from build123d import *

# Parameters (mm, degrees)
SKETCH_1_R      = 3.4
SKETCH_1_R_2    = 2.25
EXTRUDE_1_DEPTH = 4.85
EXTRUDE_START   = 0.5
SKETCH_2_R      = 2.25
SKETCH_2_R_2    = 0.5
EXTRUDE_2_DEPTH = 2
EXTRUDE_START_2 = 1.25
SKETCH_3_R      = 2.25
SKETCH_3_R_2    = 1.15
EXTRUDE_3_DEPTH = 0.9


with BuildPart() as part:
    # 草图1 → 凸台-拉伸1 (new body)
    with BuildSketch(Plane(origin=(0, 0, 0), x_dir=(1, 0, 0), z_dir=(0, 1, 0))):
        with Locations(Location((0, 0, 0), (0, 0, 270))):
            Circle(SKETCH_1_R)
        with Locations(Location((0, 0, 0), (0, 0, 270))):
            Circle(SKETCH_1_R_2, mode=Mode.SUBTRACT)
    extrude(amount=EXTRUDE_1_DEPTH)

    # 草图2 → 凸台-拉伸2 (add)
    with BuildSketch(Plane(origin=(0, 0, 0), x_dir=(1, 0, 0), z_dir=(0, 1, 0)).offset(EXTRUDE_START)):
        with BuildLine():
            Line((1.781000011, 3.395903963), (1.781000011, 6.35))
            ThreePointArc((1.781000011, 6.35), (0, 8.13100001), (-1.781000011, 6.35))
            Line((-1.781000011, 6.35), (-1.781000011, 3.342130588))
            ThreePointArc((-1.781000011, 3.342130588), (-3.786362647, -0.072496957), (-1.651758938, -3.407857144))
            Line((-1.651758938, -3.407857144), (-1.651758938, -6.35))
            ThreePointArc((-1.651758938, -6.35), (0, -8.001758939), (1.651758938, -6.35))
            Line((1.651758938, -6.35), (1.651758938, -3.407857144))
            Line((1.651758938, -3.407857144), (15.410111856, -2.130295801))
            ThreePointArc((15.410111856, -2.130295801), (17.490132215, -0.073847388), (15.557558889, 2.121744812))
            Line((15.557558889, 2.121744812), (1.781000011, 3.395903963))
        make_face()
        with Locations(Location((0, 0, 0), (0, 0, 270))):
            Circle(SKETCH_2_R, mode=Mode.SUBTRACT)
        with Locations(Location((0, -6.75, 0), (0, 0, 270))):
            Circle(SKETCH_2_R_2, mode=Mode.SUBTRACT)
        with Locations(Location((0, -4.75, 0), (0, 0, 270))):
            Circle(SKETCH_2_R_2, mode=Mode.SUBTRACT)
        with Locations(Location((15, 0, 0), (0, 0, 270))):
            Circle(SKETCH_2_R_2, mode=Mode.SUBTRACT)
        with Locations(Location((13, 0, 0), (0, 0, 270))):
            Circle(SKETCH_2_R_2, mode=Mode.SUBTRACT)
        with Locations(Location((11, 0, 0), (0, 0, 270))):
            Circle(SKETCH_2_R_2, mode=Mode.SUBTRACT)
        with Locations(Location((9, 0, 0), (0, 0, 270))):
            Circle(SKETCH_2_R_2, mode=Mode.SUBTRACT)
        with Locations(Location((7, 0, 0), (0, 0, 270))):
            Circle(SKETCH_2_R_2, mode=Mode.SUBTRACT)
        with Locations(Location((5, 0, 0), (0, 0, 270))):
            Circle(SKETCH_2_R_2, mode=Mode.SUBTRACT)
        with Locations(Location((0, 6.75, 0), (0, 0, 270))):
            Circle(SKETCH_2_R_2, mode=Mode.SUBTRACT)
        with Locations(Location((0, 4.75, 0), (0, 0, 270))):
            Circle(SKETCH_2_R_2, mode=Mode.SUBTRACT)
    extrude(amount=EXTRUDE_2_DEPTH)

    # 草图3 → 凸台-拉伸3 (add)
    with BuildSketch(Plane(origin=(0, 0, 0), x_dir=(1, 0, 0), z_dir=(0, 1, 0)).offset(EXTRUDE_START_2)):
        with Locations(Location((0, 0, 0), (0, 0, 270))):
            Circle(SKETCH_3_R)
        with Locations(Location((0, 0, 0), (0, 0, 270))):
            Circle(SKETCH_3_R_2, mode=Mode.SUBTRACT)
    extrude(amount=EXTRUDE_3_DEPTH)


solid = part.part
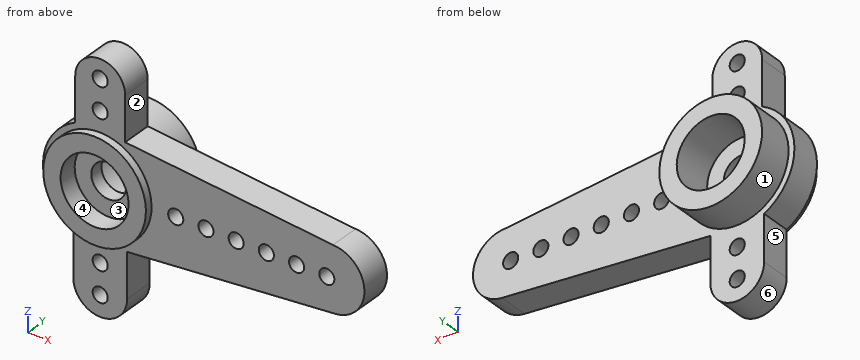
The listing builds one solid part. Answer for the finished solid, in the listing's coordinates (mm). Face numbers are marked on the shaded views. A direction names the side the tool comes from. Give positions to 0.01 mm unless a question says otherwise; leave off trailing zeros. Write each loop counter-clockwise with the first axis right and the second up, starting at its lowest first coordinate (ties: lowest second). Pieces come first, ordered by that corner, then holes. Notation, with made-up numbers: (1, 15.5) - (34, 15.5) arc R25 cw to (34, 32.5) - close; hole circle Ø3 at (39.25, -27). An arc over 180 degrees is marked (long way). Use a Markdown table: item, result.
1. Section C-C on y = 4.3 is taken. Write down the section's boundary in (x, z).
Values follow:
| item | result |
|---|---|
| outline | circle Ø6.8 at (0, 0); hole circle Ø4.5 at (0, 0) |
2. For a pull along X with two mould halves and no side action, classify the marked faces 4, 5 and 6 as released by +X, released by -X, zero draft, split by the parting line, or undercut.
Values follow:
| item | result |
|---|---|
| face 4 | undercut |
| face 5 | released by -X |
| face 6 | split by the parting line |
3. Section D-D on z = -2.75 is taken. Write down the section's boundary in (x, y).
Values follow:
| item | result |
|---|---|
| outline | (-2.6, 0.5) - (-2, 0.5) - (-2, 0) - (2, 0) - (2, 0.5) - (8.76, 0.5) - (8.76, 2.5) - (2, 2.5) - (2, 4.85) - (-2, 4.85) - (-2, 2.5) - (-2.6, 2.5) - close |
4. Find the intervals of material crossed by probe 1 along Y at (x, z) = (16.75, -1.5); probe 2 along X at (y, z) = (2.05, 4.75); probe 3 along X at (y, z) = (1, -4.75), in increasing order. Write a range as from..to.
Values follow:
| item | result |
|---|---|
| probe 1 | y = 0.5..2.5 |
| probe 2 | x = -1.65..-0.5, 0.5..1.65 |
| probe 3 | x = -1.78..-0.5, 0.5..1.78 |
5. Section A-A on z = 4.75 is taken. Write down the section's boundary in (x, y), plus the area to 3 significant figures.
Values follow:
| item | result |
|---|---|
| outline | (-1.65, 0.5) - (-0.5, 0.5) - (-0.5, 2.5) - (-1.65, 2.5) - close; (0.5, 0.5) - (1.65, 0.5) - (1.65, 2.5) - (0.5, 2.5) - close |
| area | 4.61 mm² |
6. Section B-B on x = 7.25 is taken. Write down the section's boundary in (y, z).
Values follow:
| item | result |
|---|---|
| outline | (0.5, -2.89) - (2.5, -2.89) - (2.5, -0.43) - (0.5, -0.43) - close; (0.5, 0.43) - (2.5, 0.43) - (2.5, 2.89) - (0.5, 2.89) - close |
7. Each of these flat-tipped pins is pushed along its axis until it touches: P1, Ø3, axis at x = 0, z = 0, coming from the +Y side; P2, Ø1.6, axis at y = 1, z = 5.5, coming from the +X side; P3, Ø0.6, axis at y = 2, z = -4, coming from the +X side. Where does it stop, or does it pass through?
Values follow:
| item | result |
|---|---|
| P1 | stops at y = 2.15 |
| P2 | stops at x = 1.65 |
| P3 | stops at x = 1.78 |
8. A tool of negligible diameter and unlimited length cuts with its end or side. For the marked faces 1, 2 and 3, from which of +Z, -Z, +X, -X, +Y, -Y can it reach the whole face along a straight path? Write none if from no direction.
Values follow:
| item | result |
|---|---|
| face 1 | +Y |
| face 2 | +Z, +X, +Y, -Y |
| face 3 | -Y |
